from build123d import *

# Parameters (mm, degrees)
SKICA1_W                = 300
SKICA1_H                = 20
P_IDAT_VYSUNUT_M1_DEPTH = 5
F_5_0_5_PR_M_R_D_RY1_D  = 5
F_5_0_5_PR_M_R_D_RY2_D  = 5
LINPOLE1_COUNT          = 6
LINPOLE1_PITCH          = 43.333333333


with BuildPart() as part:
    # Skica1 → Přidat vysunutím1 (new body)
    with BuildSketch(Plane.XY):
        Rectangle(SKICA1_W, SKICA1_H)
    extrude(amount=P_IDAT_VYSUNUT_M1_DEPTH)

    # Ø5.0 (5) průměr díry1 (through all)
    with Locations(Plane.XY.offset(5)):
        with Locations((-130, 0)):
            f_5_0_5_pr_m_r_d_ry1 = Hole(F_5_0_5_PR_M_R_D_RY1_D / 2)

    # Ø5.0 (5) průměr díry2 (through all)
    with Locations(Plane.XY.offset(5)):
        with Locations((130, 0)):
            Hole(F_5_0_5_PR_M_R_D_RY2_D / 2)

    # LinPole1: Ø5.0 (5) průměr díry1 ×6
    with Locations(*[(i * LINPOLE1_PITCH, 0, 0) for i in range(1, LINPOLE1_COUNT)]):
        add(f_5_0_5_pr_m_r_d_ry1, mode=Mode.SUBTRACT)


solid = part.part
Could you check a few things on this model? Use its own coordinates, in mm. Give positions to 0.01 mm unless a question says otherwise; leave off trailing zeros. Loops run counter-clockwise (first coordinate to the right, second up) from the corner with the lowest first, then second, coordinate; pieces in that order, holes last. Notation, with made-up numbers: (80.25, 47.25) -> (97.25, 47.25) arc R16 ccw to (97.25, 58.25) -> close; hole circle Ø7 at (-15.75, 45.25). An arc over 180 degrees is marked (long way). Answer as CSV lines item,"result". Start each with the question number.
(1) We'd pull the mould along Y, two halves only. Please class faces 1 (the flat face through (-2, -10, 2)), 2 (the flat face through (-2, 2, 0)), 3 (the cylindrical face through (84.3, 0.8, 2.5)), 4 (the cylindrical face through (0.54, -2.44, 2.46)): released by +Y, released by -Y, zero draft, split by the parting line, or undercut.
(2) If we section it at B-B on z = 2.7: Write out the boundary of the cut face in (x, y).
(3) If we section it at A-A on y = 0: Count the separate pieces of the cut face and the enclosed holes in it, then the cut area to 4 significant figures.
(4) If we section it at C-C on x = 130: Write out the boundary of the cut face in (y, z), then the cut area to 3 significant figures.
(5) I need wall thicknesses on probe 1 along Y at (x, z) = (0, 1); probe 2 along Y at (x, z) = (-131, 1.5). Which ranges of each line are inside material? Lowest first, please.
Computed:
1,face 1,"released by -Y"
1,face 2,"zero draft"
1,face 3,"undercut"
1,face 4,"undercut"
2,outline,"(-150, -10) -> (150, -10) -> (150, 10) -> (-150, 10) -> close; hole circle Ø5 at (-130, 0); hole circle Ø5 at (-86.67, 0); hole circle Ø5 at (-43.33, 0); hole circle Ø5 at (0, 0); hole circle Ø5 at (43.33, 0); hole circle Ø5 at (86.67, 0); hole circle Ø5 at (130, 0)"
3,separate pieces,"8"
3,enclosed holes,"0"
3,area,"1,325 mm2"
4,outline,"(-10, 0) -> (-2.5, 0) -> (-2.5, 5) -> (-10, 5) -> close; (2.5, 0) -> (10, 0) -> (10, 5) -> (2.5, 5) -> close"
4,area,"75.0 mm2"
5,probe 1,"y = -10 to -2.5, 2.5 to 10"
5,probe 2,"y = -10 to -2.29, 2.29 to 10"
